from build123d import *

# Parameters (mm, degrees)
IZIM1_R                     = 1.5
Y_KSEKLIK_EKSTR_ZYON1_DEPTH = 1.5
IZIM2_R                     = 2.5
KES_EKSTR_ZYON1_DEPTH       = 0.5


with BuildPart() as part:
    # Çizim1 → Yükseklik-Ekstrüzyon1 (new body)
    with BuildSketch(Plane.XY):
        with BuildLine():
            Line((-2.5, -13), (-2.5, -4.5))
            ThreePointArc((-2.5, -4.5), (-3.085786438, -3.085786438), (-4.5, -2.5))
            Line((-4.5, -2.5), (-13, -2.5))
            ThreePointArc((-13, -2.5), (-15.5, 0), (-13, 2.5))
            Line((-13, 2.5), (-4.5, 2.5))
            ThreePointArc((-4.5, 2.5), (-3.085786438, 3.085786438), (-2.5, 4.5))
            Line((-2.5, 4.5), (-2.5, 13))
            ThreePointArc((-2.5, 13), (0, 15.5), (2.5, 13))
            Line((2.5, 13), (2.5, 4.5))
            ThreePointArc((2.5, 4.5), (3.085786438, 3.085786438), (4.5, 2.5))
            Line((4.5, 2.5), (13, 2.5))
            ThreePointArc((13, 2.5), (15.5, 0), (13, -2.5))
            Line((13, -2.5), (4.5, -2.5))
            ThreePointArc((4.5, -2.5), (3.085786438, -3.085786438), (2.5, -4.5))
            Line((2.5, -4.5), (2.5, -13))
            ThreePointArc((2.5, -13), (0, -15.5), (-2.5, -13))
        make_face()
        with Locations((0, 13)):
            Circle(IZIM1_R, mode=Mode.SUBTRACT)
        with Locations((13, 0)):
            Circle(IZIM1_R, mode=Mode.SUBTRACT)
        with Locations((0, -13)):
            Circle(IZIM1_R, mode=Mode.SUBTRACT)
        with Locations((-13, 0)):
            Circle(IZIM1_R, mode=Mode.SUBTRACT)
    extrude(amount=Y_KSEKLIK_EKSTR_ZYON1_DEPTH)

    # Çizim2 → Kes-Ekstrüzyon1 (cut)
    with BuildSketch(Plane.XY.offset(1.5)):
        Circle(IZIM2_R)
    extrude(amount=-KES_EKSTR_ZYON1_DEPTH, mode=Mode.SUBTRACT)


solid = part.part
Input: part model. Units: mm. Frame: model coordinates. A direction names the side the tool comes from. Give positions to 0.01 mm unless a question says otherwise; leave off trailing zeros. Order: outer loops, then holes, each group sorted by start corner. A loop starts at its lowest first (then second) coordinate and runs counter-clockwise, first axis right, second up. Notation, with made-up numbers: (-39.75, 74.25) - (-33.75, 74.25) arc R6 ccw to (-33.75, 81.25) - close; hole circle Ø3 at (52, 74). An arc over 180 degrees is marked (long way). Answer as a JSON object with one key per item and string values. Group by question number.
Q1. Cut plane C-C, the plane x = 12. Output: boundary loops of the cut face in (y, z), then the cut area to 3 significant figures.
Q2. Set-up query: faces 1 (the face through (-2.5, 9, 1)), 2 (the face through (2.5, -9, 1)), 3 (the face through (2.5, 9, 1)), 4 (the face through (0, 0, 1)), 5 (the face through (-9, -2.5, 1)). Return all of +Z, -Z, +X, -X, +Y, -Y with unobstructed straight access to the full face (end or side cutting, diameter ignored); none if empty.
Q3. First-contact query: pin 1 Ø0.8 at (x, z) = (10.5, 1) entering from +Y; pin 2 Ø1.5 at (x, y) = (0, -0.5) entering from +Z. Flat tips, straight axial feed; report the tip coordinate or a pass-through.
Q4. Line query: probe 1 along Y at (x, z) = (0, 0.65); probe 2 along Y at (x, z) = (0, 1.25); probe 3 along Y at (x, z) = (-13, 0.35). Output: solid intervals per line, ascending.
Q5. Cut plane B-B, the plane z = 0.3. Output: boundary loops of the cut face in (x, y), then the cut area to 3 significant figures.
Q6. Mould query, pull axis X, two halves, no side actions, for faces 6 (the face through (11.5, 0.07, 0.74)), 7 (the face through (9, 2.5, 1)), 8 (the face through (-2.5, -9, 1)). Classes: pulls with the +X half, pulls with the -X half, needs draft (parallel to the pull), parting line crosses it, or undercut.
Q7. Cut plane A-A, the plane y = 0. Output: boundary loops of the cut face in (x, z).
Q8. Cut plane D-D, the plane x = 1. Output: boundary loops of the cut face in (y, z).
Results:
{
 "1": {"outline": "(-2.5, 0) - (-1.12, 0) - (-1.12, 1.5) - (-2.5, 1.5) - close; (1.12, 0) - (2.5, 0) - (2.5, 1.5) - (1.12, 1.5) - close", "area": "4.15 mm^2"},
 "2": {"face 1": "+Z, -Z, -X, +Y", "face 2": "+Z, -Z, +X, -Y", "face 3": "+Z, -Z, +X, +Y", "face 4": "+Z", "face 5": "+Z, -Z, -X, -Y"},
 "3": {"pin 1": "y = 2.5", "pin 2": "z = 1"},
 "4": {"probe 1": "-15.5 to -14.5, -11.5 to 11.5, 14.5 to 15.5", "probe 2": "-15.5 to -14.5, -11.5 to -2.5, 2.5 to 11.5, 14.5 to 15.5", "probe 3": "-2.5 to -1.5, 1.5 to 2.5"},
 "5": {"outline": "(-13, -2.5) - (-4.5, -2.5) arc R2 cw to (-2.5, -4.5) - (-2.5, -13) arc R2.5 ccw to (2.5, -13) - (2.5, -4.5) arc R2 cw to (4.5, -2.5) - (13, -2.5) arc R2.5 ccw to (13, 2.5) - (4.5, 2.5) arc R2 cw to (2.5, 4.5) - (2.5, 13) arc R2.5 ccw to (-2.5, 13) - (-2.5, 4.5) arc R2 cw to (-4.5, 2.5) - (-13, 2.5) arc R2.5 ccw to start; hole circle Ø3 at (-13, 0); hole circle Ø3 at (0, -13); hole circle Ø3 at (0, 13); hole circle Ø3 at (13, 0)", "area": "249 mm^2"},
 "6": {"face 6": "undercut", "face 7": "needs draft", "face 8": "pulls with the -X half"},
 "7": {"outline": "(-15.5, 0) - (-14.5, 0) - (-14.5, 1.5) - (-15.5, 1.5) - close; (-11.5, 0) - (11.5, 0) - (11.5, 1.5) - (2.5, 1.5) - (2.5, 1) - (-2.5, 1) - (-2.5, 1.5) - (-11.5, 1.5) - close; (14.5, 0) - (15.5, 0) - (15.5, 1.5) - (14.5, 1.5) - close"},
 "8": {"outline": "(-15.29, 0) - (-14.12, 0) - (-14.12, 1.5) - (-15.29, 1.5) - close; (-11.88, 0) - (11.88, 0) - (11.88, 1.5) - (2.29, 1.5) - (2.29, 1) - (-2.29, 1) - (-2.29, 1.5) - (-11.88, 1.5) - close; (14.12, 0) - (15.29, 0) - (15.29, 1.5) - (14.12, 1.5) - close"}
}
